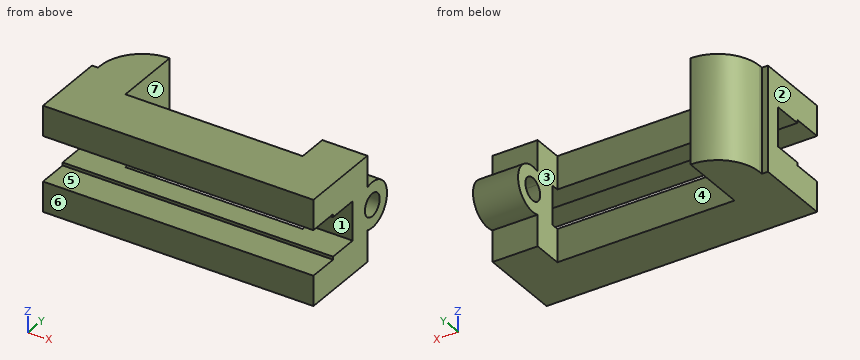
```python
from build123d import *

# Parameters (mm, degrees)
BOSS_EXTRUDE1_DEPTH = 70
CUT_EXTRUDE3_DEPTH  = 196
SKETCH5_R           = 15
SKETCH5_R_2         = 7.5
BOSS_EXTRUDE3_DEPTH = 30
CUT_EXTRUDE4_DEPTH  = 30


with BuildPart() as part:
    # Sketch1 → Boss-Extrude1 (new body)
    with BuildSketch(Plane.XY):
        with BuildLine():
            Line((0, 0), (180, 0))
            Line((180, 0), (180, 55))
            Line((180, 55), (150, 55))
            Line((150, 55), (150, 35))
            Line((150, 35), (32, 35))
            Line((32, 35), (32, 80))
            ThreePointArc((32, 80), (12.200980837, 71.799019163), (4, 52.0001))
            Line((4, 52.0001), (4, 50))
            Line((4, 50), (0, 50))
            Line((0, 50), (0, 0))
        make_face()
    extrude(amount=-BOSS_EXTRUDE1_DEPTH)

    # Sketch2 → Cut-Extrude3 (cut)
    with BuildSketch(Plane.ZY):
        Polygon((-50, 0), (-50, 20), (-48, 20), (-48, 40), (-22, 40), (-22, 20), (-20, 20), (-20, 0), align=None)
    extrude(amount=-CUT_EXTRUDE3_DEPTH, mode=Mode.SUBTRACT)

    # Sketch5 → Boss-Extrude3 (add)
    with BuildSketch(Plane.ZY.offset(-180)):
        with Locations((-35, 60)):
            Circle(SKETCH5_R)
        with Locations((-35, 60)):
            Circle(SKETCH5_R_2, mode=Mode.SUBTRACT)
    extrude(amount=BOSS_EXTRUDE3_DEPTH)

    # Sketch5_3 → Cut-Extrude4 (cut)
    with BuildSketch(Plane.ZY.offset(-180)):
        with BuildLine():
            ThreePointArc((-40.590169944, 55), (-35, 52.5), (-29.409830056, 55))
            Line((-29.409830056, 55), (-40.590169944, 55))
        make_face()
        with BuildLine():
            Line((-40.590169944, 55), (-29.409830056, 55))
            ThreePointArc((-29.409830056, 55), (-27.993707308, 57.323834327), (-27.5, 60))
            ThreePointArc((-27.5, 60), (-37.676165673, 67.006292692), (-40.590169944, 55))
        make_face()
    extrude(amount=CUT_EXTRUDE4_DEPTH, mode=Mode.SUBTRACT)


solid = part.part
```
Build history of the part. All positions in model axes, mm. Face numbers are marked on the shaded views. A direction names the side the tool comes from. Round coordinates to 2 decimals unless told otherwise and drop trailing zeros. Write each loop counter-clockwise with the first axis right and the second up, starting at its lowest first coordinate (ties: lowest second). Pieces come first, ordered by that corner, then holes.
1) Drill centre lines: probe 1 along Z at (x, y) = (163.5, 60); probe 2 along Z at (x, y) = (142.5, 24.5); probe 3 along X at (y, z) = (43.5, -31). Where is each one in solid material? Low to high.
2) Band-saw the part on A-A, the plane y = 6. List the corners of the cut face in (x, z).
3) 3-axis set-ups, long thin cutter, end or side, ignore diameter. For the marked faces 5, 6 and 7: which of +Z, -Z, +X, -X, +Y, -Y reach the whole face in a straight line?
4) Mould opens along X. For the marked faces 1, 2, 3 and 4 say: +X half, -X half, draft (parallel to the pull), parting line (faces both ways), or undercut.
5) Band-saw the part on C-C, the plane x = 121. List the corners of the cut face in (y, z), and give its area (3 significant figures).
6) Pin check, flat tips, straight feed: pin 1 (13.5 mm diameter, centred on y = 60, z = -35, fed in from -X); pin 2 (21 mm diameter, centred on x = 11, z = -29.5, fed in from -Y); pin 3 (0.6 mm diameter, centred on x = 46.5, z = -48.5, fed in from -Y); pin 4 (4 mm diameter, centred on x = 34.5, y = 46.5, fed in from -Z). Stop position of each tip, or through.
7) Band-saw the part on D-D, the plane z = -53. List the corners of the cut face in (x, y).
8) Band-saw the part on B-B, the plane z = -35. List the corners of the cut face in (x, y), and give its area (3 significant figures).
Ans:
1. probe 1: z = -50 to -42.5, -27.5 to -20
1. probe 2: z = -70 to -48, -22 to 0
1. probe 3: x = 0 to 32, 150 to 180
2. outline: (0, -70) - (180, -70) - (180, -50) - (0, -50) - close; (0, -20) - (180, -20) - (180, 0) - (0, 0) - close
3. face 5: +X, -X, -Y
3. face 6: +Z, -Z, +X, -X, -Y
3. face 7: +Z, -Z, +Y
4. face 1: draft
4. face 2: -X half
4. face 3: undercut
4. face 4: undercut
5. outline: (0, -70) - (35, -70) - (35, -48) - (20, -48) - (20, -50) - (0, -50) - close; (0, -20) - (20, -20) - (20, -22) - (35, -22) - (35, 0) - (0, 0) - close
5. area: 1,460 mm2
6. pin 1: stops at x = 4.03
6. pin 2: stops at y = 0
6. pin 3: stops at y = 20
6. pin 4: passes through
7. outline: (0, 0) - (180, 0) - (180, 55) - (150, 55) - (150, 35) - (32, 35) - (32, 80) arc R28 ccw to (4, 52) - (4, 50) - (0, 50) - close
8. outline: (0, 40) - (32, 40) - (32, 80) arc R28 ccw to (4, 52) - (4, 50) - (0, 50) - close; (150, 40) - (180, 40) - (180, 52.5) - (150, 52.5) - close; (150, 67.5) - (180, 67.5) - (180, 75) - (150, 75) - close
8. area: 1,590 mm2
